The listing builds one solid part. Answer for the finished solid, in the listing's coordinates (mm). Face numbers are marked on the shaded views. A direction names the side the tool comes from. Round coordinates to 2 decimals unless told otherwise and drop trailing zeros. Write each loop counter-clockwise with the first axis right and the second up, starting at its lowest first coordinate (ties: lowest second). Pieces come first, ordered by that corner, then holes. Notation, with made-up numbers: (-24, 21) - (28, 21) arc R24 ccw to (28, 51) - close; hole circle Ø3 at (13.5, 87). An arc over 180 degrees is marked (long way). Use a Markdown table: item, result. Add a question column.
1) Determine the mould class of the marked faces 3, 4, 5 and 6 for opening direction X: +X half, -X half, draft (parallel to the pull), parting line (faces both ways), or undercut.
2) A cutting plane is placed at A-A (y = -12.9). Give the vertices of the cut face in (x, z), then the cut area to 3 significant figures.
3) Each of these flat-tipped pins is pushed along its axis until it touches: P1, Ø1, axis at x = 21.5, y = -21.5, coming from the -Z side; P2, Ø5, axis at x = -3.5, y = -8, coming from the -Z side; P3, Ø1.3, axis at x = 22.5, y = -5.5, coming from the -Z side. Where does it stop, or does it pass through?
4) Find the intervals of material crossed by probe 1 along X at (y, z) = (-21.7, -2); probe 2 along Y at (x, z) = (-21.7, -3.2); probe 3 along X at (y, z) = (12, -5.75), in increasing order. Write a range as from..to.
5) A cutting plane is placed at C-C (z = -7.75). Give the vertices of the cut face in (x, y), then the cut area to 3 significant figures.
6) A tool of negligible diameter and unlimited length cuts with its end or side. For the marked faces 1 and 2, from which of +Z, -Z, +X, -X, +Y, -Y can it reach the whole face along a straight path? Write none if from no direction.
7) A cutting plane is placed at B-B (x = 0.5). Give the vertices of the cut face in (y, z), then the cut area to 3 significant figures.
8) A cutting plane is placed at D-D (y = 17). Give the vertices of the cut face in (x, z), then the cut area to 3 significant figures.
```python
from build123d import *

# Parameters (mm, degrees)
F0_W     = 23
F0_H     = 23
F0_R     = 8.5
F1_DEPTH = 0.6
F3_DEPTH = 9.6
F4_W     = 2.6
F4_H     = 2.6
F4_R     = 0.6
F5_DEPTH = 4.7
F6_W     = 8
F6_H     = 3
F7_DEPTH = 1.4


with BuildPart() as f1:
    # F0 (on Top) → F1 (new body, symmetric)
    with BuildSketch(Plane.XY):
        with Locations((-11.5, 11.5)):
            Rectangle(F0_W, F0_H)
        Polygon((0, -10.131208), (0, 0), (-23, 0), (-23, -23), (0, -23), (0, -15.231208), (-2.55, -15.231208), (-2.55, -10.131208), align=None)
        with Locations((-13, -12.9)):
            Circle(F0_R, mode=Mode.SUBTRACT)
        with Locations((11.5, 11.5)):
            Rectangle(F0_W, F0_H)
        Polygon((23, 0), (0, 0), (0, -10.131208), (2.55, -10.131208), (2.55, -15.231208), (0, -15.231208), (0, -23), (23, -23), align=None)
        with Locations((13, -12.9)):
            Circle(F0_R, mode=Mode.SUBTRACT)
    extrude(amount=F1_DEPTH, both=True)

    # F2 (on face) → F3 (join)
    with BuildSketch(Plane.XY.offset(0.6)):
        Polygon((-23, 23), (0, 23), (0, 24.2), (-24.2, 24.2), (-24.2, -24.2), (0, -24.2), (0, -23), (-23, -23), align=None)
        Polygon((0, 23), (23, 23), (23, -23), (0, -23), (0, -24.2), (24.2, -24.2), (24.2, 24.2), (0, 24.2), align=None)
    extrude(amount=-F3_DEPTH)

    # F4 (on face) → F5 (join)
    with BuildSketch(Plane(origin=(0, 0, -0.6), x_dir=(1, 0, 0), z_dir=(0, 0, -1))):
        with Locations((21.7, 21.7)):
            Rectangle(F4_W, F4_H)
        with Locations((21.7, 21.7)):
            Circle(F4_R, mode=Mode.SUBTRACT)
        with Locations((-21.7, 21.7)):
            Rectangle(F4_W, F4_H)
        with Locations((-21.7, 21.7)):
            Circle(F4_R, mode=Mode.SUBTRACT)
        with Locations((-21.7, 4.7)):
            Rectangle(F4_W, F4_H)
        with Locations((-21.7, 4.7)):
            Circle(F4_R, mode=Mode.SUBTRACT)
        with Locations((21.7, 4.7)):
            Rectangle(F4_W, F4_H)
        with Locations((21.7, 4.7)):
            Circle(F4_R, mode=Mode.SUBTRACT)
    extrude(amount=F5_DEPTH)

    # F6 (on face) → F7 (cut)
    with BuildSketch(Plane(origin=(-24.2, 0, 0), x_dir=(0, -1, 0), z_dir=(-1, 0, 0))):
        with Locations((-14.2, -2.3)):
            Rectangle(F6_W, F6_H)
    extrude(amount=-F7_DEPTH, mode=Mode.SUBTRACT)


solid = f1.part
```
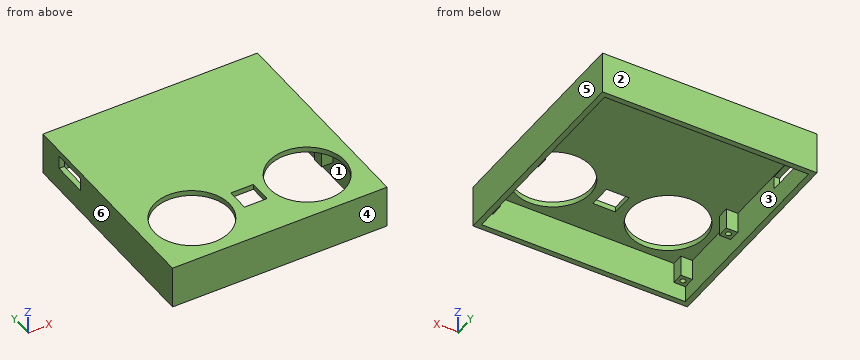
Entries:
| question | item | result |
|---|---|---|
| 1 | face 3 | undercut |
| 1 | face 4 | draft |
| 1 | face 5 | +X half |
| 1 | face 6 | -X half |
| 2 | outline | (-24.2, -9) - (-23, -9) - (-23, -0.6) - (-21.5, -0.6) - (-21.5, 0.6) - (-24.2, 0.6) - close; (-4.5, -0.6) - (-2.55, -0.6) - (-2.55, 0.6) - (-4.5, 0.6) - close; (2.55, -0.6) - (4.5, -0.6) - (4.5, 0.6) - (2.55, 0.6) - close; (21.5, -0.6) - (23, -0.6) - (23, -9) - (24.2, -9) - (24.2, 0.6) - (21.5, 0.6) - close |
| 2 | area | 31.3 mm² |
| 3 | P1 | stops at z = -5.3 |
| 3 | P2 | stops at z = -0.6 |
| 3 | P3 | stops at z = -9 |
| 4 | probe 1 | x = -24.2..-22.3, -21.1..-20.4, 20.4..21.1, 22.3..24.2 |
| 4 | probe 2 | y = -24.2..-22.3, -21.1..-20.4, -6..-5.3, -4.1..-3.4, 23..24.2 |
| 4 | probe 3 | x = -24.2..-23, 23..24.2 |
| 5 | outline | (-24.2, -24.2) - (24.2, -24.2) - (24.2, 24.2) - (-24.2, 24.2) - close; hole (-23, -23) - (23, -23) - (23, 23) - (-23, 23) - close |
| 5 | area | 227 mm² |
| 6 | face 1 | -Z |
| 6 | face 2 | +Z, -Z, +X, -X, +Y |
| 7 | outline | (-24.2, -9) - (-23, -9) - (-23, -0.6) - (-15.23, -0.6) - (-15.23, 0.6) - (-24.2, 0.6) - close; (-10.13, -0.6) - (23, -0.6) - (23, -9) - (24.2, -9) - (24.2, 0.6) - (-10.13, 0.6) - close |
| 7 | area | 72.1 mm² |
| 8 | outline | (-24.2, -9) - (-23, -9) - (-23, -3.8) - (-24.2, -3.8) - close; (-24.2, -0.8) - (-23, -0.8) - (-23, -0.6) - (23, -0.6) - (23, -9) - (24.2, -9) - (24.2, 0.6) - (-24.2, 0.6) - close |
| 8 | area | 74.6 mm² |
